from build123d import *

# Parameters (mm, degrees)
F0_W      = 63.5
F0_H      = 63.5
F0_W_2    = 50.8
F0_H_2    = 50.8
F1_DEPTH  = 165.1
F3_R      = 6.35
F4_DEPTH  = 25.4
F6_DEPTH  = 25.4
F7_R      = 6.35
F8_DEPTH  = 63.501
F9_W      = 145.7979530096
F9_H      = 377.9422044754
F9_W_2    = 50.8
F9_H_2    = 292.1
F10_DEPTH = 63.5
F11_W     = 97.6704657078
F11_H     = 338.8985395432
F12_DEPTH = 57.151
F13_R     = 11.43
F13_R_2   = 6.35
F14_DEPTH = 6.35
F15_W     = 170.8157360554
F15_H     = 347.1174836159
F16_DEPTH = 25.4


# Not quite as in the source:
# - ends of sketch curves that miss each other by under 0.0002 mm in the source are joined


with BuildPart() as f1:
    # F0 (on Top) → F1 (new body, symmetric)
    with BuildSketch(Plane.XY):
        Rectangle(F0_W, F0_H)
        Rectangle(F0_W_2, F0_H_2, mode=Mode.SUBTRACT)
    extrude(amount=F1_DEPTH, both=True)

    # F3 (on face) → F4 (cut)
    with BuildSketch(Plane.YZ.offset(31.75)):
        with Locations((0, 146.05)):
            Circle(F3_R)
        with BuildLine():
            ThreePointArc((10.1385245046, 129.1766616857), (14.6288058895, 132.8781640138), (17.8406687878, 137.7307595176))
            ThreePointArc((17.8406687878, 137.7307595176), (19.4934269332, 143.3103775076), (19.4426449846, 149.1294124443))
            ThreePointArc((19.4426449846, 149.1294124443), (15.0835370951, 152.2964897102), (11.9164598293, 147.9373818207))
            ThreePointArc((11.9164598293, 147.9373818207), (11.9475842494, 144.3708765369), (10.9346034506, 140.9511106721))
            ThreePointArc((10.9346034506, 140.9511106721), (8.9660423194, 137.9769392343), (6.2139343738, 135.708276517))
            ThreePointArc((6.2139343738, 135.708276517), (4.9104220235, 130.4801740359), (10.1385245046, 129.1766616857))
        make_face()
        with BuildLine():
            ThreePointArc((-10.1385245046, 129.1766616857), (-4.9104220235, 130.4801740359), (-6.2139343738, 135.708276517))
            ThreePointArc((-6.2139343738, 135.708276517), (-8.9660423194, 137.9769392343), (-10.9346034506, 140.9511106721))
            ThreePointArc((-10.9346034506, 140.9511106721), (-11.9475842494, 144.3708765369), (-11.9164598293, 147.9373818207))
            ThreePointArc((-11.9164598293, 147.9373818207), (-15.0835370951, 152.2964897102), (-19.4426449846, 149.1294124443))
            ThreePointArc((-19.4426449846, 149.1294124443), (-19.4934269332, 143.3103775076), (-17.8406687878, 137.7307595176))
            ThreePointArc((-17.8406687878, 137.7307595176), (-14.6288058895, 132.8781640138), (-10.1385245046, 129.1766616857))
        make_face()
    extrude(amount=-F4_DEPTH, mode=Mode.SUBTRACT)

    # F5 (on face) → F6 (cut)
    with BuildSketch(Plane(origin=(-31.75, 0, 0), x_dir=(0, -1, 0), z_dir=(-1, 0, 0))):
        with BuildLine():
            ThreePointArc((-3.0785410886, 140.4961648597), (3.2228686048, 140.5786548312), (6.35, 146.05))
            ThreePointArc((6.35, 146.05), (-3.2228686048, 151.5213451688), (-3.0785410886, 140.4961648597))
        make_face()
        with BuildLine():
            ThreePointArc((-5.7913527214, 132.1654121492), (-6.0549491708, 133.1322727306), (-6.7727903948, 133.8315626913))
            ThreePointArc((-6.7727903948, 133.8315626913), (-9.3377562721, 131.1985515677), (-5.7913527214, 132.1654121492))
        make_face()
        with BuildLine():
            ThreePointArc((3.1226517792, 134.3961049058), (0.4285749428, 129.7298269458), (5.0948529028, 127.0357501095))
            ThreePointArc((5.0948529028, 127.0357501095), (17.8406687878, 137.7307595176), (17.8406687878, 154.3692404824))
            ThreePointArc((17.8406687878, 154.3692404824), (12.777460542, 156.2120975737), (10.9346034506, 151.1488893279))
            ThreePointArc((10.9346034506, 151.1488893279), (10.9346034506, 140.9511106721), (3.1226517792, 134.3961049058))
        make_face()
    extrude(amount=-F6_DEPTH, mode=Mode.SUBTRACT)

    # F7 (on face) → F8 (cut, through all)
    with BuildSketch(Plane.YZ.offset(31.75)):
        with BuildLine():
            ThreePointArc((-8.89, 107.949999693), (-15.239999693, 101.6), (-8.89, 95.250000307))
            ThreePointArc((-8.89, 95.250000307), (3.81, 82.55), (-8.89, 69.85))
            ThreePointArc((-8.89, 69.85), (-15.239999693, 63.5), (-8.89, 57.150000307))
            ThreePointArc((-8.89, 57.150000307), (16.509999693, 82.55), (-8.89, 107.949999693))
        make_face()
        with BuildLine():
            ThreePointArc((8.89, 3.07e-07), (15.239999693, 6.35), (8.89, 12.699999693))
            ThreePointArc((8.89, 12.699999693), (-3.81, 25.4), (8.89, 38.1))
            ThreePointArc((8.89, 38.1), (15.24, 44.45), (8.89, 50.8))
            ThreePointArc((8.89, 50.8), (-16.509999693, 25.4), (8.89, 3.07e-07))
        make_face()
        with BuildLine():
            ThreePointArc((-8.89, -6.350000307), (-15.239999693, -12.7), (-8.89, -19.049999693))
            ThreePointArc((-8.89, -19.049999693), (3.81, -31.75), (-8.89, -44.45))
            ThreePointArc((-8.89, -44.45), (-15.239999693, -50.8), (-8.89, -57.149999693))
            ThreePointArc((-8.89, -57.149999693), (16.509999693, -31.75), (-8.89, -6.350000307))
        make_face()
        with BuildLine():
            ThreePointArc((8.89, -114.299999693), (15.239999693, -107.95), (8.89, -101.600000307))
            ThreePointArc((8.89, -101.600000307), (-3.81, -88.9), (8.89, -76.2))
            ThreePointArc((8.89, -76.2), (15.24, -69.85), (8.89, -63.5))
            ThreePointArc((8.89, -63.5), (-16.509999693, -88.9), (8.89, -114.299999693))
        make_face()
        with Locations((-8.89, 82.55)):
            Circle(F7_R)
        with Locations((8.89, 25.4)):
            Circle(F7_R)
        with Locations((8.89, -88.9)):
            Circle(F7_R)
        with Locations((-8.89, -31.75)):
            Circle(F7_R)
    extrude(amount=-F8_DEPTH, mode=Mode.SUBTRACT)

    # F9 (on face) → F10 (cut, symmetric)
    with BuildSketch(Plane(origin=(25.4, 0, 0), x_dir=(0, -1, 0), z_dir=(-1, 0, 0))):
        Rectangle(F9_W, F9_H)
        with Locations((0, 19.05)):
            Rectangle(F9_W_2, F9_H_2, mode=Mode.SUBTRACT)
    extrude(amount=F10_DEPTH, both=True, mode=Mode.SUBTRACT)

    # F11 (on face) → F12 (cut, through all)
    with BuildSketch(Plane.YZ.offset(-25.4)):
        Rectangle(F11_W, F11_H)
    extrude(amount=F12_DEPTH, mode=Mode.SUBTRACT)

    # F13 (on face) → F14 (join)
    with BuildSketch(Plane(origin=(-31.75, 0, 0), x_dir=(0, -1, 0), z_dir=(-1, 0, 0))):
        with Locations((0, 146.05)):
            Circle(F13_R)
        with Locations((0, 146.05)):
            Circle(F13_R_2, mode=Mode.SUBTRACT)
    extrude(amount=F14_DEPTH)

    # F15 (on face) → F16 (cut)
    with BuildSketch(Plane(origin=(-31.75, 0, 0), x_dir=(0, -1, 0), z_dir=(-1, 0, 0))):
        Rectangle(F15_W, F15_H)
    extrude(amount=-F16_DEPTH, mode=Mode.SUBTRACT)


solid = f1.part
Model file for the job. Use its own axes, mm. Give positions to 0.01 mm unless a question says otherwise; leave off trailing zeros. Order: outer loops, then holes, each group sorted by start corner. A loop starts at its lowest first (then second) coordinate and runs counter-clockwise, first axis right, second up. Notation, with made-up numbers: (-8.75, -14) - (22.25, -14) arc R18 cw to (22.25, -5) - close; hole circle Ø10 at (-10.5, 14.25). An arc over 180 degrees is marked (long way). Write item = value, one per line. Start each with the question number.
1. Probe line 1 along Z through (x, y) = (-36.25, 0); line 2 along Z through (x, y) = (-36.5, 2.75); line 3 along Y through (x, z) = (-35, 146.75). List the from-to ranges inside material, lowest first.
2. Cut at A-A, the plane y = 0. List the corners of the cut face in (x, z), and give its area (3 significant figures).
3. Cut at D-D, the plane y = -9.5. List the corners of the cut face in (x, z), and give its area (3 significant figures).
4. Cut at B-B, the plane z = 146.05. List the corners of the cut face in (x, y).
5. Drop a flat-ended pin along its axis: P1, Ø1.5, axis at x = -37, y = 7, coming from the -Z side. Give the stop position or say it passes through.
6. Two-plate mould, pull along Z, no slides. Class faces 1 (the flat face through (-38.1, -5, 141)), 2 (the cylindrical face through (-34.881, 2.478, 134.892)), 3 (the cylindrical face through (-34.881, -5.866, 143.618)): pulls with the +Z half, pulls with the -Z half, needs draft (parallel to the pull), parting line crosses it, or undercut.
7. Cut at C-C, the plane x = -33. List the corners of the cut face in (y, z).
Taken from the geometry:
q1.line_1 = 134.62 to 139.7, 152.4 to 157.48
q1.line_2 = 134.96 to 140.33, 151.77 to 157.14
q1.line_3 = -11.41 to -6.31, 6.31 to 11.41
q2.outline = (-38.1, 134.62) - (-31.75, 134.62) - (-31.75, 139.7) - (-38.1, 139.7) - close; (-38.1, 152.4) - (-31.75, 152.4) - (-31.75, 157.48) - (-38.1, 157.48) - close
q2.area = 64.5 mm²
q3.outline = (-38.1, 139.69) - (-31.75, 139.69) - (-31.75, 152.41) - (-38.1, 152.41) - close
q3.area = 80.7 mm²
q4.outline = (-38.1, -11.43) - (-31.75, -11.43) - (-31.75, -6.35) - (-38.1, -6.35) - close; (-38.1, 6.35) - (-31.75, 6.35) - (-31.75, 11.43) - (-38.1, 11.43) - close
q5.P1 = 136.48
q6.face_1 = needs draft
q6.face_2 = parting line crosses it
q6.face_3 = undercut
q7.outline = circle Ø22.86 at (0, 146.05); hole circle Ø12.7 at (0, 146.05)
